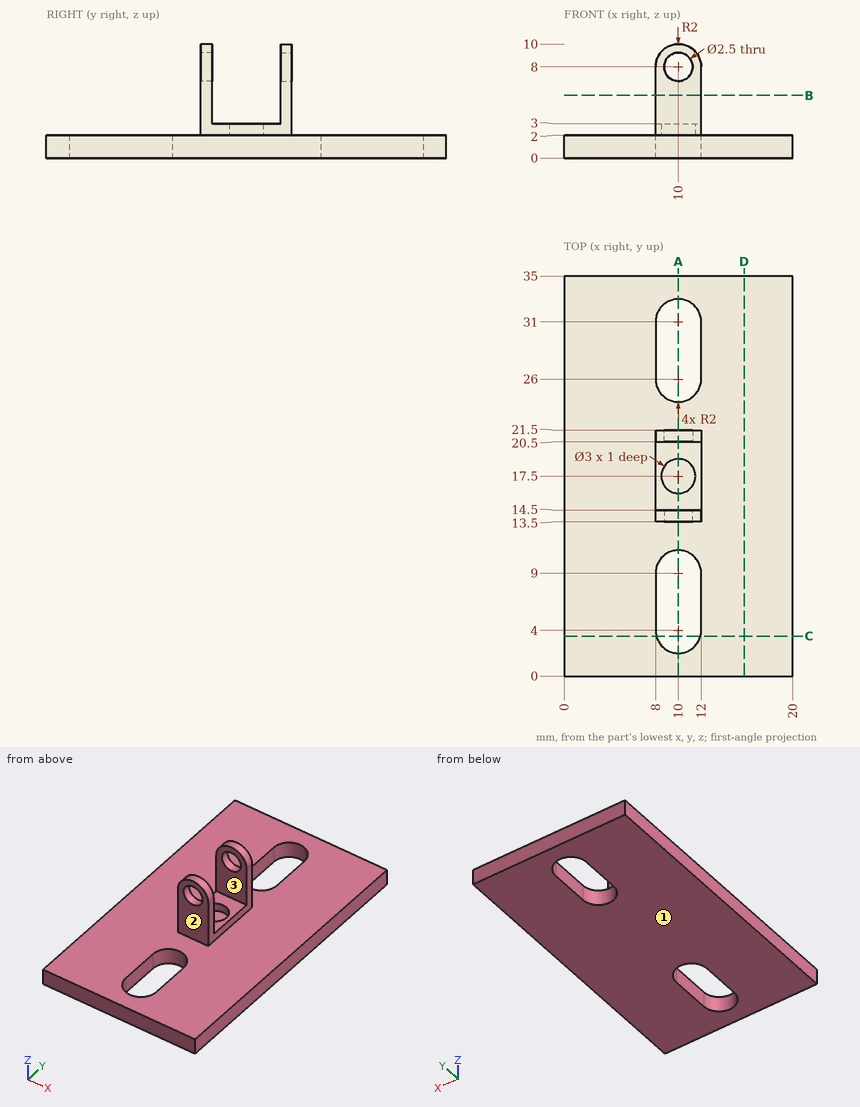
Source: three-view drawing plus pictorial views. Frame: mm from the lowest corner of the part. A direction names the side the tool comes from. Round coordinates to 2 decimals unless told otherwise and drop trailing zeros. Loops run counter-clockwise (first coordinate to the right, second up) from the corner with the lowest first, then second, coordinate; pieces in that order, holes last. Notation, with made-up numbers: M -37.5,33 L -14.5,33 A20 cw -14.5,60 Z; hole C 54,59.25 d8. An arc over 180 degrees is marked long. Put each result on its own line as item: value. Start each with the question number.
(1) Material intervals for line 1 along Y through (x, z) = (10, 2.65); line 2 along X through (y, z) = (20.8, 8); line 3 along X through (y, z) = (29, 0.5), sorted ascending. Write a range as [from, to].
(2) Section query D-D (x = 15.75). Return loops of the section in (y, z), then the cut area to 3 significant figures.
(3) Section query B-B (z = 5.5). Return loops of the section in (x, y).
(4) Set-up query: the marked faces 1, 2 and 3. Return all of +Z, -Z, +X, -X, +Y, -Y with unobstructed straight access to the full face (end or side cutting, diameter ignored); none if empty.
(5) Section query C-C (y = 3.5). Return loops of the section in (x, z), then the cut area to 3 significant figures.
(6) Section query A-A (x = 10). State how many separate pieces and enclosed holes the cut face has, then the cut area to 3 significant figures.
(7) Contact query for flat-ended pins moving along their axis: pin 1 Ø1.2 at (x, z) = (9, 7) entering from -Y; pin 2 Ø1.5 at (y, z) = (14, 5.5) entering from -X; pin 3 Ø2 at (x, y) = (11, 16.5) entering from +Z. Output: stop coordinate, or through.
Findings below:
1. line 1: y = [13.5, 16], [19, 21.5]
1. line 2: x = [8, 8.75], [11.25, 12]
1. line 3: x = [0, 8], [12, 20]
2. outline: M 0,0 L 35,0 L 35,2 L 0,2 Z
2. area: 70.0 mm2
3. outline: M 8,13.5 L 12,13.5 L 12,14.5 L 8,14.5 Z; M 8,20.5 L 12,20.5 L 12,21.5 L 8,21.5 Z
4. face 1: -Z, +X, -X, +Y, -Y
4. face 2: +Z, +X, -X, -Y
4. face 3: +Z, +X, -X
5. outline: M 0,0 L 8.06,0 L 8.06,2 L 0,2 Z; M 11.94,0 L 20,0 L 20,2 L 11.94,2 Z
5. area: 32.3 mm2
6. separate pieces: 5
6. enclosed holes: 0
6. area: 48.0 mm2
7. pin 1: stops at y = 13.5
7. pin 2: stops at x = 8
7. pin 3: stops at z = 3
